Source: CAD feature listing. Evaluate the final solid. Frame: model axes, mm. Face numbers are marked on the shaded views. A direction names the side the tool comes from. Coordinates: 2 decimals unless noted, no trailing zeros. Order: outer loops, then holes, each group sorted by start corner. A loop starts at its lowest first (then second) coordinate and runs counter-clockwise, first axis right, second up.
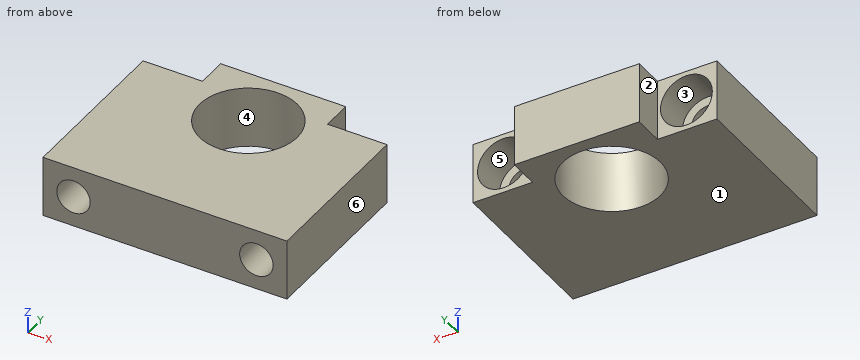
Autodesk Inventor part; units mm, degrees
ref_plane "bf_1_XY" through (0, 0, 0) normal (0, 0, 1) x (1, 0, 0)
ref_plane "bf_1_YZ" through (0, 0, 0) normal (1, 0, 0) x (0, 1, 0)
ref_plane "bf_1_ZX" through (0, 0, 0) normal (0, 1, 0) x (0, 0, 1)
sketch "Sketch_1" plane through (0, 0, 0) normal (0, 0, 1) x (1, 0, 0)
  line L0 (20, 10) -> (39.5, 10)
  line L1 (39.5, 10) -> (39.5, -20)
  line L2 (20, 10) -> (20, 20)
  line L3 (20, 20) -> (-21, 20)
  line L4 (-21, 20) -> (-21, 10)
  line L5 (-21, 10) -> (-40.5, 10)
  line L6 (-40.5, 10) -> (-40.5, -20)
  line L7 (-40.5, -20) -> (39.5, -20)
  dimension "d29" = 19.5
  dimension "d42" = 10
  dimension "d43" = 41
  dimension "d44" = 19.5
  dimension "d54" = 30
  dimension "d55" = 0
extrude "Extrusion1" add sketch "Sketch_1" against normal blind 20
sketch "Sketch4" plane through (0, 0, 0) normal (0, 0, 1) x (1, 0, 0)
  point P0 (0, 0)
hole "Hole3" at (0, 0, 0) direction (0, 0, -1) diameter 32 depth 20
ref_plane "bf_1_XY" through (0, 0, 0) normal (0, 0, 1) x (1, 0, 0)
ref_plane "bf_1_YZ" through (0, 0, 0) normal (1, 0, 0) x (0, 1, 0)
ref_plane "bf_1_ZX" through (0, 0, 0) normal (0, 1, 0) x (0, 0, 1)
ref_plane "bf_2x_XY" through (0, 0, -10) normal (0, 0, 1) x (1, 0, 0)
ref_plane "bf_2x_YZ" through (0, 0, -10) normal (1, 0, 0) x (0, 1, 0)
ref_plane "bf_2x_ZX" through (0, 0, -10) normal (0, 1, 0) x (0, 0, 1)
sketch "Sketch6" plane through (20, 10, 0) normal (0, 1, 0) x (1, 0, 0)
  line L0 (0, 0) -> (19.5, 0)
  line L1 (19.5, 0) -> (9.5, 0)
  line L2 (9.5, 0) -> (9.5, 10)
  line L3 (-60.5, 0) -> (-41, 0)
  line L4 (-60.5, 0) -> (-50.5, 0)
  line L5 (-50.5, 0) -> (-50.5, 10)
  dimension "d45" = 10
  dimension "d46" = 10
  dimension "d47" = 10
hole "Hole4" at (29.5, 10, -10) at (-30.5, 10, -10) direction (0, -1, 0) diameter 11 end through all counterbore diameter 17 counterbore depth 12
sketch "Sketch9" plane through (-40.5, -20, 0) normal (0, -1, 0) x (1, 0, 0)
  line L0 (80, -20) -> (60.5, -20)
  line L1 (0, 0) -> (0, -20)
  line L2 (80, -20) -> (0, -20)
  line L3 (0, -20) -> (0, 0)
  line L4 (0, 0) -> (80, 0)
  line L5 (80, 0) -> (80, -20)
  circle A0 centre (70, -10) radius 5.5
  circle A1 centre (70, -10) radius 5.5
  circle A2 centre (10, -10) radius 5.5
  circle A3 centre (10, -10) radius 5.5
  point P0 (40.5, 0)
  dimension "d48" = 11
  dimension "d49" = 11
extrude "Extrusion2" add sketch "Sketch9" along normal blind 25
properties part number "BF 15 Part1"
1. Section query A-A on y = 0. Return loops of the section in (x, z), plus the area to 3 significant figures.
Findings:
outline: (-40.5, -20) - (-16, -20) - (-16, 0) - (-40.5, 0) - close; (16, -20) - (39.5, -20) - (39.5, 0) - (16, 0) - close; hole circle Ø17 at (-30.5, -10); hole circle Ø17 at (29.5, -10)
area: 506 mm2
2. Section query D-D on x = -30.5. Return loops of the section in (y, z).
Findings:
outline: (-45, -20) - (10, -20) - (10, -18.5) - (-2, -18.5) - (-2, -15.5) - (-45, -15.5) - close; (-45, -4.5) - (-2, -4.5) - (-2, -1.5) - (10, -1.5) - (10, 0) - (-45, 0) - close
3. Section query B-B on z = -10. Return loops of the section in (x, y).
Findings:
outline: (-40.5, -45) - (-36, -45) - (-36, -2) - (-39, -2) - (-39, 10) - (-40.5, 10) - close; (-25, -45) - (24, -45) - (24, -2) - (21, -2) - (21, 10) - (20, 10) - (20, 20) - (-21, 20) - (-21, 10) - (-22, 10) - (-22, -2) - (-25, -2) - close; (35, -45) - (39.5, -45) - (39.5, 10) - (38, 10) - (38, -2) - (35, -2) - close; hole circle Ø32 at (0, 0)
4. Ray query, line 1 (X direction, y = -35.5, z = -10); line 2 (Z direction, x = 29.5, y = 1); line 3 (X direction, y = -24, z = -6). Return the intervals inside material, ascending.
Findings:
line 1: x = -40.5 to -36, -25 to 24, 35 to 39.5
line 2: z = -20 to -18.5, -1.5 to 0
line 3: x = -40.5 to -34.27, -26.73 to 25.73, 33.27 to 39.5
5. Draft query along X for the marked faces 1, 2, 3 and 4. Return one class per face: released by +X, released by -X, zero draft, split by the parting line, or undercut.
Findings:
face 1: zero draft
face 2: released by -X
face 3: undercut
face 4: undercut
6. Access query for the marked faces 5 and 6. Directions: +Z, -Z, +X, -X, +Y, -Y. A direction counts if a zero-diameter tool reaches every point of the face in a straight line with its end or side. Return the directions, or none.
Findings:
face 5: +Y
face 6: +Z, -Z, +X, +Y, -Y
7. Pin query (flat end, axial travel): P1, Ø5, axis at y = 13.5, z = -11, coming from the +X side; P2, Ø5, axis at x = 31, z = -6, coming from the +Y side. Return the tip coordinate at first contact, or that it passes through.
Findings:
P1: stops at x = 20
P2: stops at y = -2
8. Section query C-C on x = 0. Return loops of the section in (y, z), plus the area to 3 significant figures.
Findings:
outline: (-45, -20) - (-16, -20) - (-16, 0) - (-45, 0) - close; (16, -20) - (20, -20) - (20, 0) - (16, 0) - close
area: 660 mm2
